from build123d import *

# Parameters (mm, degrees)
SKETCH1_W           = 25
SKETCH1_H           = 25
BOSS_EXTRUDE1_DEPTH = 8
SKETCH2_R           = 2
SKETCH2_R_2         = 0.75
SKETCH2_R_3         = 2.5
CUT_EXTRUDE1_DEPTH  = 8
CUT_EXTRUDE2_DEPTH  = 4


with BuildPart() as part:
    # Sketch1 → Boss-Extrude1 (new body)
    with BuildSketch(Plane(origin=(0, 0, 0), x_dir=(1, 0, 0), z_dir=(0, 1, 0))):
        Rectangle(SKETCH1_W, SKETCH1_H)
    extrude(amount=BOSS_EXTRUDE1_DEPTH)

    # Sketch2 → Cut-Extrude1 (cut)
    with BuildSketch(Plane(origin=(0, 8, 0), x_dir=(1, 0, 0), z_dir=(0, 1, 0))):
        with Locations(Location((-5.191248411, 6.850045341, 0), (0, 0, 270))):
            Circle(SKETCH2_R)
        with Locations(Location((6.814693369, 7.491872418, 0), (0, 0, 270))):
            Circle(SKETCH2_R_2)
        with Locations(Location((-4.247385064, -5.417775614, 0), (0, 0, 270))):
            Circle(SKETCH2_R_3)
    extrude(amount=-CUT_EXTRUDE1_DEPTH, mode=Mode.SUBTRACT)

    # Sketch3 → Cut-Extrude2 (cut)
    with BuildSketch(Plane(origin=(0, 8, 0), x_dir=(1, 0, 0), z_dir=(0, 1, 0))):
        Polygon((-0.572446257, 6.850045341), (-2.881847334, 10.850045341), (-7.500649488, 10.850045341), (-9.810050565, 6.850045341), (-7.500649488, 2.850045341), (-2.881847334, 2.850045341), align=None)
        Polygon((0.948767359, -5.417775614), (-1.649308852, -0.917775614), (-6.845461275, -0.917775614), (-9.443537486, -5.417775614), (-6.845461275, -9.917775614), (-1.649308852, -9.917775614), align=None)
    extrude(amount=-CUT_EXTRUDE2_DEPTH, mode=Mode.SUBTRACT)


solid = part.part
Build history of the part. All positions in model axes, mm. A direction names the side the tool comes from. Coordinates: 2 decimals unless noted, no trailing zeros. Order: outer loops, then holes, each group sorted by start corner. A loop starts at its lowest first (then second) coordinate and runs counter-clockwise, first axis right, second up. Notation, with made-up numbers: (-39, -16) -> (-32, -16) arc R23 cw to (-32, 12) -> close; hole circle Ø10 at (-25, 0). An arc over 180 degrees is marked (long way). One line per item, written item: value.
(1) Slice it at D-D, the plane y = 7. List the corners of the cut face in (x, z).
Checked values:
outline: (-12.5, -12.5) -> (12.5, -12.5) -> (12.5, 12.5) -> (-12.5, 12.5) -> close; hole (-9.81, -6.85) -> (-7.5, -10.85) -> (-2.88, -10.85) -> (-0.57, -6.85) -> (-2.88, -2.85) -> (-7.5, -2.85) -> close; hole (-9.44, 5.42) -> (-6.85, 0.92) -> (-1.65, 0.92) -> (0.95, 5.42) -> (-1.65, 9.92) -> (-6.85, 9.92) -> close; hole circle Ø1.5 at (6.81, -7.49)
(2) Slice it at C-C, the plane x = -8. List the corners of the cut face in (y, z).
Checked values:
outline: (0, -12.5) -> (8, -12.5) -> (8, -9.99) -> (4, -9.99) -> (4, -3.71) -> (8, -3.71) -> (8, 2.92) -> (4, 2.92) -> (4, 7.92) -> (8, 7.92) -> (8, 12.5) -> (0, 12.5) -> close
(3) Probe line 1 (Z direction, x = -4, y = 7.25); line 2 (Z direction, x = -4, y = 1.5); line 3 (Z direction, x = -9.5, y = 6). List the from-to ranges inside material, lowest first. Write a range as [from, to].
Checked values:
line 1: [-12.5, -10.85], [-2.85, 0.92], [9.92, 12.5]
line 2: [-12.5, -8.46], [-5.24, 2.93], [7.91, 12.5]
line 3: [-12.5, -7.39], [-6.31, 12.5]
(4) Slice it at A-A, the plane z = 5. List the corners of the cut face in (x, y), plus the area to 3 significant figures.
Checked values:
outline: (-12.5, 0) -> (-6.71, 0) -> (-6.71, 4) -> (-9.2, 4) -> (-9.2, 8) -> (-12.5, 8) -> close; (-1.78, 0) -> (12.5, 0) -> (12.5, 8) -> (0.71, 8) -> (0.71, 4) -> (-1.78, 4) -> close
area: 141 mm2
(5) Slice it at B-B, the plane y = 3.25. List the corners of the cut face in (x, z), plus the area to 3 significant figures.
Checked values:
outline: (-12.5, -12.5) -> (12.5, -12.5) -> (12.5, 12.5) -> (-12.5, 12.5) -> close; hole circle Ø4 at (-5.19, -6.85); hole circle Ø5 at (-4.25, 5.42); hole circle Ø1.5 at (6.81, -7.49)
area: 591 mm2
(6) Tool access for faces 1 (the flat face through (-8.16, 6.03, 7.64)), 2 (the cylindrical face through (-7, 2, -6)): list every direction of +Z, -Z, +X, -X, +Y, -Y with a clear straight run to the whole face (end or side of a thin tool).
Checked values:
face 1: +Y
face 2: +Y, -Y
(7) Drop flat-ended pins along their axis: pin 1 Ø7 at (x, z) = (-4, 3.5) entering from +Y; pin 2 Ø4.5 at (x, z) = (-5.19, -6.85) entering from +Y; pin 3 Ø1.2 at (x, z) = (6.81, -7.49) entering from +Y. Give the stop position or say it passes through.
Checked values:
pin 1: y = 8
pin 2: y = 4
pin 3: through
(8) Mould opens along X. For faces 3 (the flat face through (-12.5, 4, 0)), 4 (the flat face through (12.5, 4, 0)), 5 (the flat face through (0, 0, 0)), 6 (the flat face through (-4, 4, -9)) say: pulls with the +X half, pulls with the -X half, needs draft (parallel to the pull), parting line crosses it, or undercut.
Checked values:
face 3: pulls with the -X half
face 4: pulls with the +X half
face 5: needs draft
face 6: undercut
